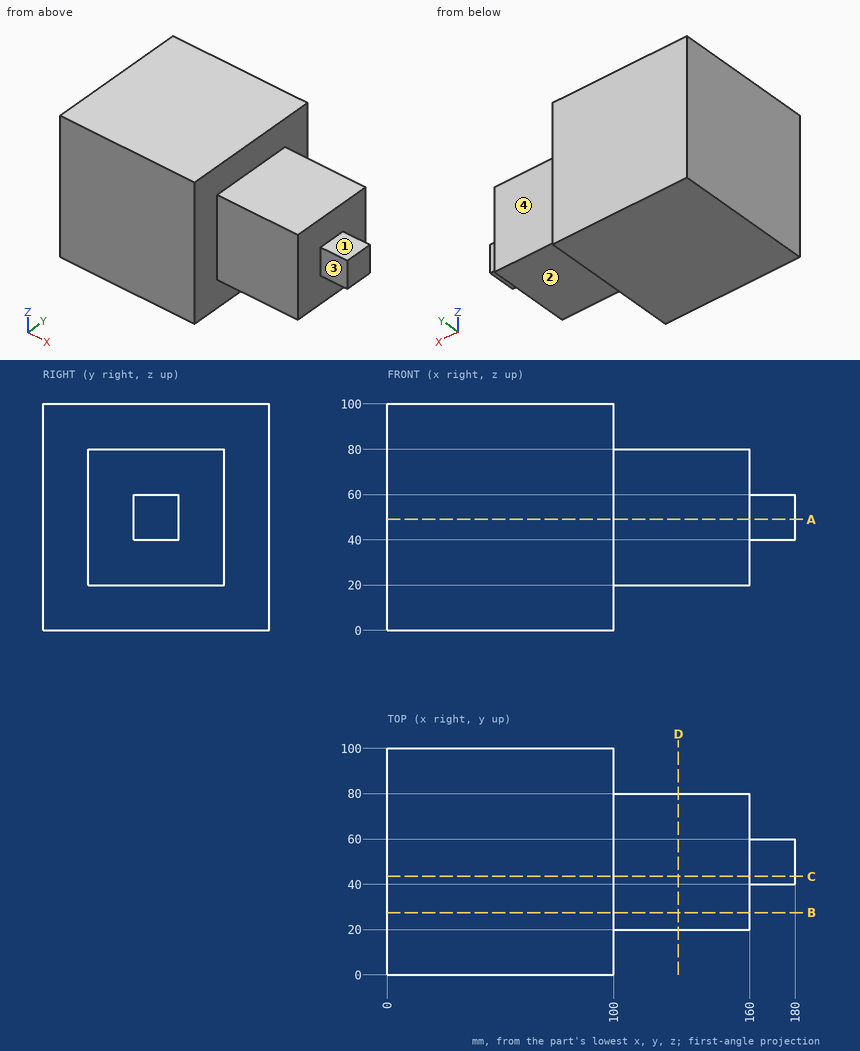
Check sheet for the drawn part. Datum: minimum x, y, z corner. Units: mm. A direction names the side the tool comes from. Give positions to 0.01 mm unless a question says otherwise; leave off trailing zeros. Order: outer loops, then holes, each group sorted by start corner. A loop starts at its lowest first (then second) coordinate and runs counter-clockwise, first axis right, second up. Notation, with made-up numbers: (40.25, 24.5) -> (78.25, 24.5) arc R13 ccw to (78.25, 43.5) -> close; hole circle Ø6 at (25, -24). An arc over 180 degrees is marked (long way). Answer as CSV lines item,"result".
Q1. Sectioned sample at D-D on x = 128.5. Record the cut outline in (y, z).
Solutions:
outline,"(20, 20) -> (80, 20) -> (80, 80) -> (20, 80) -> close"
Q2. Sectioned sample at B-B on y = 27.5. Record the cut outline in (x, z).
Solutions:
outline,"(0, 0) -> (100, 0) -> (100, 20) -> (160, 20) -> (160, 80) -> (100, 80) -> (100, 100) -> (0, 100) -> close"
Q3. Scan lines: probe 1 along Y at (x, z) = (109, 43); probe 2 along X at (y, z) = (11.5, 4.5). Record each from-to range of solid material in increasing order.
Solutions:
probe 1,"y = 20 to 80"
probe 2,"x = 0 to 100"
Q4. Access from +Z, -Z, +X, -X, +Y, -Y to the whole of each face (thin tool, end or side, straight path). Record for the marked faces 1, 2, 3 and 4.
Solutions:
face 1,"+Z, +X, +Y, -Y"
face 2,"-Z, +X, +Y, -Y"
face 3,"+Z, -Z, +X, -Y"
face 4,"+Z, -Z, +X, +Y"
Q5. Depth check by flat-ended pin: pin 1 (10 mm diameter, centred on x = 173.5, z = 47, fed in from +Y); pin 2 (16 mm diameter, centred on x = 172.5, y = 47.5, fed in from +Z); pin 3 (18 mm diameter, centred on x = 118, z = 39.5, fed in from -Y). Enter the tip coordinate at first touch or a pass-through.
Solutions:
pin 1,"stops at y = 60"
pin 2,"stops at z = 60"
pin 3,"stops at y = 20"
Q6. Sectioned sample at A-A on z = 49. Record the cut outline in (x, y), plus the area to 3 significant figures.
Solutions:
outline,"(0, 0) -> (100, 0) -> (100, 20) -> (160, 20) -> (160, 40) -> (180, 40) -> (180, 60) -> (160, 60) -> (160, 80) -> (100, 80) -> (100, 100) -> (0, 100) -> close"
area,"14,000 mm²"
